```python
from build123d import *

# Parameters (mm, degrees)
F1_DEPTH = 1.5
F2_DEPTH = 42


with BuildPart() as f1:
    # F0 (on Front) → F1 (new body)
    with BuildSketch(Plane.XZ):
        with BuildLine():
            Line((32.5, 8), (-32.5, 8))
            ThreePointArc((-32.5, 8), (-40.5, 0), (-32.5, -8))
            Line((-32.5, -8), (32.5, -8))
            ThreePointArc((32.5, -8), (40.5, 0), (32.5, 8))
        make_face()
        with BuildLine():
            Line((32.5, 8.5), (-32.5, 8.5))
            Line((-32.5, 8.5), (-32.5, 8))
            Line((-32.5, 8), (32.5, 8))
            ThreePointArc((32.5, 8), (40.5, 0), (32.5, -8))
            Line((32.5, -8), (32.5, -8.5))
            ThreePointArc((32.5, -8.5), (41, 0), (32.5, 8.5))
        make_face()
        with BuildLine():
            Line((-32.5, 8), (-32.5, 8.5))
            ThreePointArc((-32.5, 8.5), (-41, 0), (-32.5, -8.5))
            Line((-32.5, -8.5), (32.5, -8.5))
            Line((32.5, -8.5), (32.5, -8))
            Line((32.5, -8), (-32.5, -8))
            ThreePointArc((-32.5, -8), (-40.5, 0), (-32.5, 8))
        make_face()
    extrude(amount=F1_DEPTH)

    # F0 (on Front) → F2 (join)
    with BuildSketch(Plane.XZ):
        with BuildLine():
            Line((32.5, 9.9), (-32.5, 9.9))
            Line((-32.5, 9.9), (-32.5, 8.5))
            Line((-32.5, 8.5), (32.5, 8.5))
            ThreePointArc((32.5, 8.5), (41, 0), (32.5, -8.5))
            Line((32.5, -8.5), (32.5, -9.9))
            ThreePointArc((32.5, -9.9), (42.4, 0), (32.5, 9.9))
        make_face()
        with BuildLine():
            Line((-32.5, 8.5), (-32.5, 9.9))
            ThreePointArc((-32.5, 9.9), (-42.4, 0), (-32.5, -9.9))
            Line((-32.5, -9.9), (32.5, -9.9))
            Line((32.5, -9.9), (32.5, -8.5))
            Line((32.5, -8.5), (-32.5, -8.5))
            ThreePointArc((-32.5, -8.5), (-41, 0), (-32.5, 8.5))
        make_face()
    extrude(amount=F2_DEPTH)


solid = f1.part
```
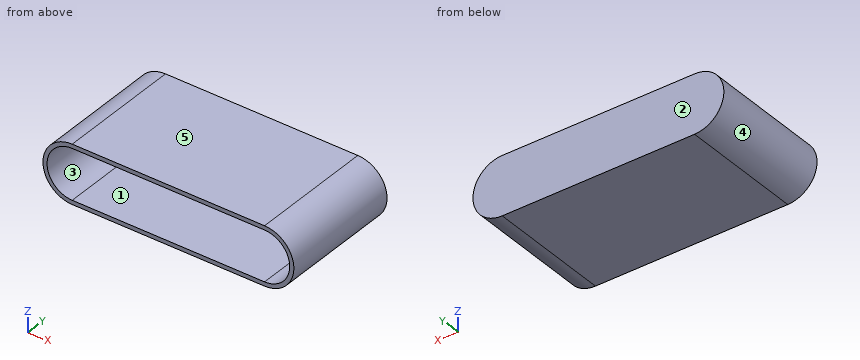
Part model, mm, in its own coordinate system. Face numbers are marked on the shaded views. A direction names the side the tool comes from. Coordinates: 2 decimals unless noted, no trailing zeros. Order: outer loops, then holes, each group sorted by start corner. A loop starts at its lowest first (then second) coordinate and runs counter-clockwise, first axis right, second up. Notation, with made-up numbers: (69.25, 70) -> (116.25, 70) arc R35 ccw to (116.25, 102) -> close; hole circle Ø5 at (17.25, -14). An arc over 180 degrees is marked (long way). Put each result on its own line as item: value. Start each with the question number.
(1) Probe line 1 along Z through (x, y) = (26, -37); line 2 along Y through (x, z) = (10, -4.25); line 3 along X through (y, z) = (-33.5, -7). List the from-to ranges inside material, lowest first. Write a range as [from, to].
(2) Band-saw the part on A-A (z = 0). Give the cut face in (x, y).
(3) Mould opens along Z. For the marked faces 3, 4 and 5 say: pulls with the +Z half, pulls with the -Z half, needs draft (parallel to the pull), parting line crosses it, or undercut.
(4) Band-saw the part on B-B (y = -31). Give the cut face in (x, z).
(5) Pin check, flat tips, straight feed: pin 1 Ø2 at (x, z) = (12.5, -1.5) entering from -Y; pin 2 Ø1 at (x, z) = (-22.5, 3.5) entering from +Y; pin 3 Ø1.5 at (y, z) = (-19, -1.5) entering from +X. Stop position of each tip, or through.
(6) Band-saw the part on C-C (x = 1.5). Give the cut face in (y, z).
(7) Which spindle directions (+Z, -Z, +X, -X, +Y, -Y) get a long thin tool onto all of the face, cutting with end or side? Do the marked faces 1 and 2. Say none if no direction does.
Determined:
1. line 1: z = [-9.9, -8.5], [8.5, 9.9]
1. line 2: y = [-1.5, 0]
1. line 3: x = [-39.5, -37.32], [37.32, 39.5]
2. outline: (-42.4, -42) -> (-41, -42) -> (-41, -1.5) -> (41, -1.5) -> (41, -42) -> (42.4, -42) -> (42.4, 0) -> (-42.4, 0) -> close
3. face 3: undercut
3. face 4: parting line crosses it
3. face 5: pulls with the +Z half
4. outline: (-32.5, -9.9) -> (32.5, -9.9) arc R9.9 ccw to (32.5, 9.9) -> (-32.5, 9.9) arc R9.9 ccw to start; hole (-32.5, -8.5) -> (32.5, -8.5) arc R8.5 ccw to (32.5, 8.5) -> (-32.5, 8.5) arc R8.5 ccw to start
5. pin 1: stops at y = -1.5
5. pin 2: stops at y = 0
5. pin 3: stops at x = 42.37
6. outline: (-42, -9.9) -> (0, -9.9) -> (0, 9.9) -> (-42, 9.9) -> (-42, 8.5) -> (-1.5, 8.5) -> (-1.5, -8.5) -> (-42, -8.5) -> close
7. face 1: -Y
7. face 2: +Z, -Z, +X, -X, +Y
